```python
from build123d import *

# Parameters (mm, degrees)
CHAMFER1_SIZE = 0.0254
FILLET1_R     = 0.79375


with BuildPart() as part:
    # Sketch3 → Revolve1 (revolve)
    with BuildSketch(Plane(origin=(0, 0, 0), x_dir=(0, 0, -1), z_dir=(1, 0, 0)), mode=Mode.PRIVATE) as revolve1_sk:
        Polygon((-3.96875, 2.38125), (3.96875, 2.38125), (3.96875, 6.35), (0.29694964, 6.35), (0.106342336, 10.715625), (0, 11.1125), (-0.106342336, 10.715625), (-0.29694964, 6.35), (-3.96875, 6.35), align=None)
    revolve(revolve1_sk.sketch.rotate(Axis((0, 0, 3.96875), (0, 0, -1)), 180), axis=Axis((0, 0, 3.96875), (0, 0, -1)))

    # Chamfer1
    chamfer1_edges = [part.edges().sort_by_distance(p)[0] for p in [
        (0, 2.38125, 3.96875),
        (0, 6.35, 3.96875),
        (0, 6.35, -3.96875),
        (0, 2.38125, -3.96875),
    ]]
    chamfer(chamfer1_edges, length=CHAMFER1_SIZE)

    # Fillet1
    fillet1_edges = [part.edges().sort_by_distance(p)[0] for p in [
        (0, 6.35, 0.29694964),
        (0, 6.35, -0.29694964),
    ]]
    fillet(fillet1_edges, radius=FILLET1_R)


solid = part.part
```
Part model, mm, in its own coordinate system. A direction names the side the tool comes from. Round coordinates to 2 decimals unless told otherwise and drop trailing zeros. Loops run counter-clockwise (first coordinate to the right, second up) from the corner with the lowest first, then second, coordinate; pieces in that order, holes last.
1. Drill centre lines: line 1 along X through (y, z) = (0, -1.75); line 2 along X through (y, z) = (-0.75, -2); line 3 along Y through (x, z) = (1.25, -1.5). Where is each one in solid material? Low to high.
Solutions:
line 1: x = -6.35 to -2.38, 2.38 to 6.35
line 2: x = -6.31 to -2.26, 2.26 to 6.31
line 3: y = -6.23 to -2.03, 2.03 to 6.23
2. 3-axis set-ups, long thin cutter, end or side, ignore diameter. For faces 1 (the face through (6.507, -3.385, -0.254)), 2 (the face through (-1.907, -6.057, 2.52)): which of +Z, -Z, +X, -X, +Y, -Y reach the whole face in a straight line?
Solutions:
face 1: -Z
face 2: +Z
3. Flat gauge pins, fed straight in: pin 1 (6 mm diameter, centred on x = 0, y = 0, fed in from +Z); pin 2 (1 mm diameter, centred on x = -3, z = -2, fed in from +Y); pin 3 (3 mm diameter, centred on x = -5.5, z = -3, fed in from -Y). Where does each tip first touch, or does it go through?
Solutions:
pin 1: stops at z = 3.97
pin 2: stops at y = 5.84
pin 3: stops at y = -4.93
4. Two-plate mould, pull along X, no slides. Class faces 3 (the face through (-1.907, -6.057, -2.48)), 4 (the face through (3, 0, -3.969)), 5 (the face through (2.325, 0.516, -0.055)): pulls with the +X half, pulls with the -X half, needs draft (parallel to the pull), parting line crosses it, or undercut.
Solutions:
face 3: parting line crosses it
face 4: needs draft
face 5: undercut
5. Slice it at A-A (z = -3.5). Give the cut face in (x, y).
Solutions:
outline: circle Ø12.7 at (0, 0); hole circle Ø4.76 at (0, 0)
